Input: part model. Units: mm. Frame: model coordinates. Face numbers are marked on the shaded views. A direction names the side the tool comes from. Give positions to 0.01 mm unless a question says otherwise; leave off trailing zeros. Loops run counter-clockwise (first coordinate to the right, second up) from the corner with the lowest first, then second, coordinate; pieces in that order, holes last. Notation, with made-up numbers: (36, 23.25) -> (67, 23.25) arc R22 ccw to (67, 35.25) -> close; hole circle Ø9 at (12, -19.5). An arc over 180 degrees is marked (long way). Answer as a JSON object with one key per item and string values.
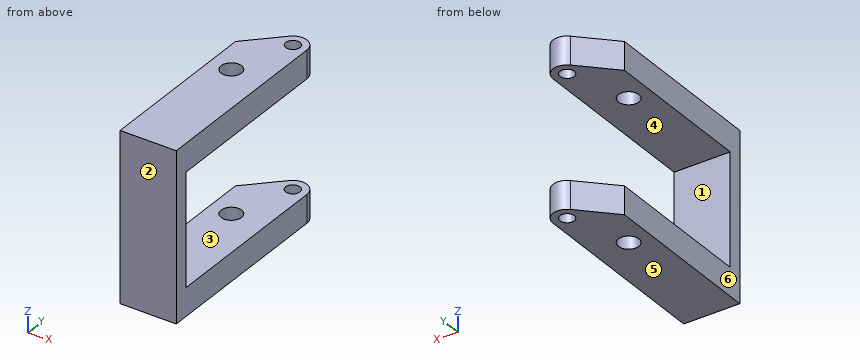
```python
from build123d import *

# Parameters (mm, degrees)
F0_R     = 4.654194
F1_DEPTH = 76.2
F2_R     = 6.35
F3_W     = 97.109872
F3_H     = 25.4
F4_DEPTH = 25.401
F5_R     = 3.2385
F6_DEPTH = 76.201


with BuildPart() as f1:
    # F0 (on Top) → F1 (new body)
    with BuildSketch(Plane.XY):
        Polygon((0, 76.2), (0, 0), (25.4, 0), (25.4, 101.6), align=None)
        with Locations((9.850098, 59.060045)):
            Circle(F0_R, mode=Mode.SUBTRACT)
    extrude(amount=-F1_DEPTH)

    # F2
    f2_edges = [f1.edges().sort_by_distance(p)[0] for p in [
        (25.4, 101.6, -38.1),
    ]]
    fillet(f2_edges, radius=F2_R)

    # F3 (on face) → F4 (cut, through all)
    with BuildSketch(Plane(origin=(0, 0, 0), x_dir=(0, -1, 0), z_dir=(-1, 0, 0))):
        with Locations((-54.904936, -50.8)):
            Rectangle(F3_W, F3_H)
        with Locations((-54.904936, -25.4)):
            Rectangle(F3_W, F3_H)
    extrude(amount=-F4_DEPTH, mode=Mode.SUBTRACT)

    # F5 (on face) → F6 (cut, through all)
    with BuildSketch(Plane(origin=(0, 0, -76.2), x_dir=(1, 0, 0), z_dir=(0, 0, -1))):
        with Locations((19.05, -86.269744)):
            Circle(F5_R)
    extrude(amount=-F6_DEPTH, mode=Mode.SUBTRACT)


solid = f1.part
```
Q1. Draft query along Z for the marked faces 3, 4, 5 and 6. Return one class per face: +Z half, -Z half, draft (parallel to the pull), parting line (faces both ways), or undercut.
Evaluation:
{"face 3": "undercut", "face 4": "undercut", "face 5": "-Z half", "face 6": "draft"}
Q2. Access query for the marked faces 1 and 2. Directions: +Z, -Z, +X, -X, +Y, -Y. A direction counts if a zero-diameter tool reaches every point of the face in a straight line with its end or side. Return the directions, or none.
Evaluation:
{"face 1": "+X, -X, +Y", "face 2": "+Z, -Z, +X, -X, -Y"}
Q3. Section B-B, the plane y = 38.5. Return the cut outline in (x, z), then the cut area to 3 significant figures.
Evaluation:
{"outline": "(0, -76.2) -> (25.4, -76.2) -> (25.4, -63.5) -> (0, -63.5) -> close; (0, -12.7) -> (25.4, -12.7) -> (25.4, 0) -> (0, 0) -> close", "area": "645 mm2"}
Q4. Pin query (flat end, axial travel): pin 1 (12.5 mm diameter, centred on x = 15, z = -38.5, fed in from +Y); pin 2 (10 mm diameter, centred on y = 51, z = -20, fed in from -X). Return the tip coordinate at first contact, or that it passes through.
Evaluation:
{"pin 1": "stops at y = 6.35", "pin 2": "passes through"}
Q5. Section D-D, the plane x = 24.25. Return the cut outline in (y, z).
Evaluation:
{"outline": "(0, -76.2) -> (89.91, -76.2) -> (89.91, -63.5) -> (6.35, -63.5) -> (6.35, -12.7) -> (89.91, -12.7) -> (89.91, 0) -> (0, 0) -> close"}
Q6. Section C-C, the plane z = -68. Return the cut outline in (x, y).
Evaluation:
{"outline": "(0, 0) -> (25.4, 0) -> (25.4, 86.27) arc R6.35 ccw to (14.56, 90.76) -> (0, 76.2) -> close; hole circle Ø9.31 at (9.85, 59.06); hole circle Ø6.48 at (19.05, 86.27)"}
Q7. Section A-A, the plane x = 19.05. Return the cut outline in (y, z).
Evaluation:
{"outline": "(0, -76.2) -> (83.03, -76.2) -> (83.03, -63.5) -> (6.35, -63.5) -> (6.35, -12.7) -> (83.03, -12.7) -> (83.03, 0) -> (0, 0) -> close; (89.51, -76.2) -> (92.62, -76.2) -> (92.62, -63.5) -> (89.51, -63.5) -> close; (89.51, -12.7) -> (92.62, -12.7) -> (92.62, 0) -> (89.51, 0) -> close"}
Q8. Ray query, line 1 along Z through (x, y) = (22.5, 24); line 2 along Y through (x, z) = (19.05, -68.75); line 3 along Y through (x, z) = (17, -27). Return the intervals inside material, ascending.
Evaluation:
{"line 1": "z = -76.2 to -63.5, -12.7 to 0", "line 2": "y = 0 to 83.03, 89.51 to 92.62", "line 3": "y = 0 to 6.35"}
